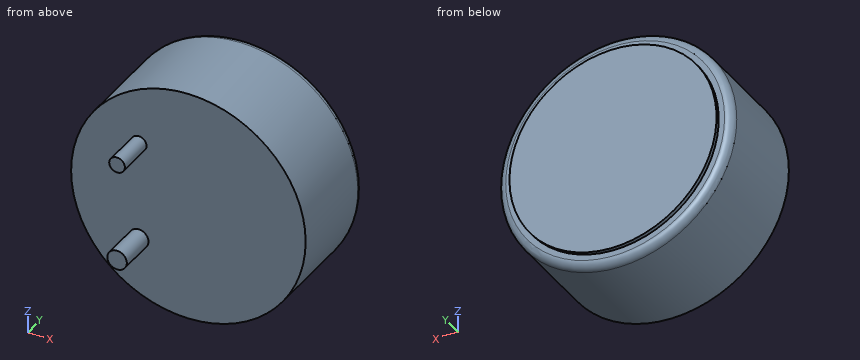
from build123d import *

# Parameters (mm, degrees)
SKETCH1_R           = 3
BOSS_EXTRUDE1_DEPTH = 2.6
FILLET1_R           = 0.2
SKETCH2_R           = 2.65
BOSS_EXTRUDE2_DEPTH = 0.1
SKETCH3_R           = 0.2
SKETCH3_R_2         = 0.25
BOSS_EXTRUDE3_DEPTH = 1


with BuildPart() as part:
    # Sketch1 → Boss-Extrude1 (new body)
    with BuildSketch(Plane(origin=(0, 0, 0), x_dir=(1, 0, 0), z_dir=(0, 1, 0))):
        Circle(SKETCH1_R)
    extrude(amount=BOSS_EXTRUDE1_DEPTH)

    # Fillet1
    fillet1_edges = [part.edges().sort_by_distance(p)[0] for p in [
        (-3, 2.6, 0),
    ]]
    fillet(fillet1_edges, radius=FILLET1_R)

    # Sketch2 → Boss-Extrude2 (add)
    with BuildSketch(Plane(origin=(0, 2.6, 0), x_dir=(1, 0, 0), z_dir=(0, 1, 0))):
        Circle(SKETCH2_R)
    extrude(amount=BOSS_EXTRUDE2_DEPTH)

    # Sketch3 → Boss-Extrude3 (add)
    with BuildSketch(Plane.XZ):
        with Locations((-1.27, 1.27)):
            Circle(SKETCH3_R)
        with Locations((-1.27, -1.27)):
            Circle(SKETCH3_R_2)
    extrude(amount=BOSS_EXTRUDE3_DEPTH)


solid = part.part
Read the model definition and answer for the solid it produces. Units are mm, in the model's axes. Round coordinates to 2 decimals unless told otherwise and drop trailing zeros. Write each loop counter-clockwise with the first axis right and the second up, starting at its lowest first coordinate (ties: lowest second). Pieces come first, ordered by that corner, then holes.
1. The part is cut by section A-A, the plane z = 0. Determine the outline of the cut face in (x, y), then the cut area to 3 significant figures.
2. Given pin 1 Ø1 at (x, z) = (0.5, -2.5) entering from -Y; pin 2 Ø2 at (y, z) = (1, -1.5) entering from -X, each flat-ended and moving along its own axis, determine where each tip first touches the part or whether it passes through.
3. Straight lines are drawn through the part: L1, parallel to Y at x = 1, z = 2.5; L2, parallel to Y at x = 2.25, z = 1; L3, parallel to X at y = 0.45, z = -2.25. For each, find the intervals that lie inside material, in ascending order.
4. The part is cut by section D-D, the plane y = 0.9. Determine the outline of the cut face in (x, z).
5. The part is cut by section B-B, the plane x = 0. Determine the outline of the cut face in (y, z).
6. The part is cut by section C-C, the plane y = -0.55. Determine the outline of the cut face in (x, z).
Values:
1. outline: (-3, 0) - (3, 0) - (3, 2.4) arc R0.2 ccw to (2.8, 2.6) - (2.65, 2.6) - (2.65, 2.7) - (-2.65, 2.7) - (-2.65, 2.6) - (-2.8, 2.6) arc R0.2 ccw to (-3, 2.4) - close
1. area: 16.1 mm2
2. pin 1: stops at y = 0
2. pin 2: stops at x = -2.96
3. L1: y = 0 to 2.6
3. L2: y = 0 to 2.7
3. L3: x = -1.98 to 1.98
4. outline: circle Ø6 at (0, 0)
5. outline: (0, -3) - (2.4, -3) arc R0.2 ccw to (2.6, -2.8) - (2.6, -2.65) - (2.7, -2.65) - (2.7, 2.65) - (2.6, 2.65) - (2.6, 2.8) arc R0.2 ccw to (2.4, 3) - (0, 3) - close
6. outline: circle Ø0.5 at (-1.27, -1.27); circle Ø0.4 at (-1.27, 1.27)
